Geometry: final body of the model. Coordinates: model frame, mm. Round coordinates to 2 decimals unless told otherwise and drop trailing zeros. Order: outer loops, then holes, each group sorted by start corner. A loop starts at its lowest first (then second) coordinate and runs counter-clockwise, first axis right, second up. Notation, with made-up numbers: M -31,-26.75 L 24,-26.75 A21 ccw 24,-4.75 Z; hole C -29.75,68 d5. An arc over 180 degrees is marked long. Put each result on its own line as item: value. Start each with the question number.
1) Section B-B, the plane x = -97. Return loops of the section in (y, z), then the cut area to 3 significant figures.
2) Section A-A, the plane y = 51.5. Return loops of the section in (x, z), then the cut area to 3 significant figures.
3) Material intervals for probe 1 along Y at (x, z) = (185, 1.8); probe 2 along Y at (x, z) = (-168.5, 1.1); probe 3 along Y at (x, z) = (-125, 1.7), sorted ascending. Write a range as [from, to].
4) Section C-C, the plane z = 1.4. Count the separate pieces of the cut face and the enclosed holes in it, then the cut area to 3 significant figures.
from build123d import *

# Parameters (mm, degrees)
SKETCH1_W           = 390
SKETCH1_H           = 227
SKETCH1_W_2         = 328
SKETCH1_H_2         = 207
BOSS_EXTRUDE1_DEPTH = 3
SKETCH2_R           = 1.5
CUT_EXTRUDE1_DEPTH  = 4
SKETCH3_R           = 1.5
CUT_EXTRUDE2_DEPTH  = 4


with BuildPart() as part:
    # Sketch1 → Boss-Extrude1 (new body)
    with BuildSketch(Plane.XY):
        Rectangle(SKETCH1_W, SKETCH1_H)
        Rectangle(SKETCH1_W_2, SKETCH1_H_2, mode=Mode.SUBTRACT)
    extrude(amount=BOSS_EXTRUDE1_DEPTH)

    # Sketch2 → Cut-Extrude1 (cut, through all)
    with BuildSketch(Plane.XY.offset(3)):
        with Locations((-185, 63.5)):
            Circle(SKETCH2_R)
        with Locations((-185, -6.5)):
            Circle(SKETCH2_R)
        with Locations((185, -6.5)):
            Circle(SKETCH2_R)
        with Locations((185, 63.5)):
            Circle(SKETCH2_R)
    extrude(amount=-CUT_EXTRUDE1_DEPTH, mode=Mode.SUBTRACT)

    # Sketch3 → Cut-Extrude2 (cut, through all)
    with BuildSketch(Plane.XY.offset(3)):
        with Locations((-169, 60)):
            Circle(SKETCH3_R)
        with Locations((-169, -60)):
            Circle(SKETCH3_R)
        with Locations((169, -60)):
            Circle(SKETCH3_R)
        with Locations((169, 60)):
            Circle(SKETCH3_R)
    extrude(amount=-CUT_EXTRUDE2_DEPTH, mode=Mode.SUBTRACT)


solid = part.part
Result sheet:
1. outline: M -113.5,0 L -103.5,0 L -103.5,3 L -113.5,3 Z; M 103.5,0 L 113.5,0 L 113.5,3 L 103.5,3 Z
1. area: 60.0 mm2
2. outline: M -195,0 L -164,0 L -164,3 L -195,3 Z; M 164,0 L 195,0 L 195,3 L 164,3 Z
2. area: 186 mm2
3. probe 1: y = [-113.5, -8], [-5, 62], [65, 113.5]
3. probe 2: y = [-113.5, -61.41], [-58.59, 58.59], [61.41, 113.5]
3. probe 3: y = [-113.5, -103.5], [103.5, 113.5]
4. separate pieces: 1
4. enclosed holes: 9
4. area: 20,600 mm2
